Autodesk Inventor part; units mm, degrees
ref_plane "YZ Plane" through (0, 0, 0) normal (1, 0, 0) x (0, 1, 0)
ref_plane "XZ Plane" through (0, 0, 0) normal (0, 1, 0) x (-1, 0, 0)
ref_plane "XY Plane" through (0, 0, 0) normal (0, 0, 1) x (1, 0, 0)
sketch "Sketch1" plane through (0, 0, 0) normal (0, 1, 0) x (-1, 0, 0)
  line L0 (-6.5, -2.5) -> (6.5, -2.5)
  line L1 (6.5, -2.5) -> (6.5, 2.5)
  line L2 (6.5, 2.5) -> (-6.5, 2.5)
  line L3 (-6.5, 2.5) -> (-6.5, -2.5)
  line L4 (-6.5, -2.5) -> (6.5, 2.5) construction
  line L5 (6.5, -2.5) -> (-6.5, 2.5) construction
  point P0 (0, 0)
  dimension "d0" = 13
  dimension "d1" = 5
extrude "Extrusion1" add sketch "Sketch1" along normal blind 70.4
sketch "Sketch2" plane through (0, 70.4, 0) normal (0, 1, 0) x (1, 0, 0)
  line L0 (6.5, 2.5) -> (6.5, -2.5)
  line L1 (6.5, -2.5) -> (-6.5, -2.5)
  line L2 (-6.5, -2.5) -> (-6.5, 2.5)
  line L3 (-6.5, 2.5) -> (6.5, 2.5)
  line L4 (-6.5, -2.5) -> (6.5, -2.5)
  line L5 (6.5, -2.5) -> (6.5, 15.2)
  line L6 (6.5, 15.2) -> (-6.5, 15.2)
  line L7 (-6.5, 15.2) -> (-6.5, -2.5)
  point P0 (0, 0)
  dimension "d4" = 17.7
extrude "Extrusion2" add sketch "Sketch2" against normal blind 5 contours L3 L7 L6 L5
fillet "Fillet1" radius 6.5 2 edges at (6.5, 0, 0) (-6.5, 0, 0)
sketch "Sketch3" plane through (6.5, 65.4, -2.5) normal (0, 0, -1) x (-1, 0, 0)
  arc A0 (0, -58.9) -> (13, -58.9) centre (6.5, -58.9) ccw
  line L0 (0, -58.9) -> (0, 0)
  line L1 (0, 0) -> (0, 5)
  line L2 (0, 5) -> (13, 5)
  line L3 (13, 5) -> (13, 0)
  line L4 (13, 0) -> (13, -58.9)
  line L5 (13, 0) -> (0, 0)
  circle A1 centre (6.5, -58.9) radius 6.5
  point P0 (6.5, -65.4)
extrude "Extrusion3" add sketch "Sketch3" along normal blind 5 contours A1 A0
sketch "Sketch4" plane through (0, 70.4, 0) normal (0, 1, 0) x (1, 0, 0)
  line L0 (6.5, -2.5) -> (-6.5, -2.5)
  line L1 (-6.5, -2.5) -> (-6.5, 15.2)
  line L2 (-6.5, 15.2) -> (6.5, 15.2)
  line L3 (6.5, 15.2) -> (6.5, -2.5)
  line L4 (6.5, -2.5) -> (-6.5, -2.5)
  line L5 (-6.5, -2.5) -> (-6.5, 15.2)
  line L6 (-6.5, 15.2) -> (6.5, 15.2)
  line L7 (6.5, 15.2) -> (6.5, -2.5)
  line L8 (-6.5, 2.5) -> (6.5, 2.5)
  circle A0 centre (0, 8.85) radius 2
  point P0 (0, 0)
  dimension "d10" = 4
  dimension "d11" = 6.35
  dimension "d12" = 6.5
extrude "Extrusion4" cut sketch "Sketch4" against normal up to surface (5 mm away) contours A0
properties part number "terminal_mount_front"
Part model, mm, in its own coordinate system. A direction names the side the tool comes from. Coordinates: 2 decimals unless noted, no trailing zeros. Write each loop counter-clockwise with the first axis right and the second up, starting at its lowest first coordinate (ties: lowest second). Pieces come first, ordered by that corner, then holes. Notation, with made-up numbers: (39.5, 66) - (76.5, 66) arc R30 ccw to (76.5, 90) - close; hole circle Ø1 at (67.25, 28). An arc over 180 degrees is marked (long way). Put each result on its own line as item: value.
1. Band-saw the part on D-D (y = 58.5). Write the cut outline in (x, z), then the cut area to 3 significant figures.
Final values:
outline: (-6.5, -2.5) - (6.5, -2.5) - (6.5, 2.5) - (-6.5, 2.5) - close
area: 65.0 mm²
2. 3-axis set-ups, long thin cutter, end or side, ignore diameter. For faces 1 (the flat face through (-2, 65.4, -10)), 2 (the cylindrical face through (-0.26, 67.935, -10.833)), 3 (the flat face through (0, 7, -7.5)): which of +Z, -Z, +X, -X, +Y, -Y reach the whole face in a straight line?
Final values:
face 1: -Z, +X, -X
face 2: +Y
face 3: -Z, +X, -X, -Y
3. Band-saw the part on B-B (z = -4.75). Write the cut outline in (x, y).
Final values:
outline: circle Ø13 at (0, 6.5); (-6.5, 65.4) - (6.5, 65.4) - (6.5, 70.4) - (-6.5, 70.4) - close
4. Flat gauge pins, fed straight in: pin 1 Ø2 at (x, z) = (0, -11.5) entering from -Y; pin 2 Ø4 at (x, z) = (-3, -6) entering from -Y. Where does each tip first touch, or does it go through?
Final values:
pin 1: stops at y = 65.4
pin 2: stops at y = 0.08
5. Probe line 1 along Z through (x, y) = (0, 68.8); line 2 along X through (y, z) = (66.45, -8.85); line 3 along Z through (x, y) = (-5.5, 50). List the from-to ranges inside material, lowest first. Write a range as [from, to].
Final values:
line 1: z = [-15.2, -10.85], [-6.85, 2.5]
line 2: x = [-6.5, -2], [2, 6.5]
line 3: z = [-2.5, 2.5]
6. Band-saw the part on A-A (z = -8.85). Write the cut outline in (x, y).
Final values:
outline: (-6.5, 65.4) - (-2, 65.4) - (-2, 70.4) - (-6.5, 70.4) - close; (2, 65.4) - (6.5, 65.4) - (6.5, 70.4) - (2, 70.4) - close
7. Two-plate mould, pull along Y, no slides. Class faces 4 (the flat face through (0, 70.4, -6)), 5 (the flat face through (-6.5, 43, -2)), 6 (the flat face through (0, 36, -2.5)): +Y half, -Y half, draft (parallel to the pull), parting line (faces both ways), or undercut.
Final values:
face 4: +Y half
face 5: draft
face 6: undercut
8. Band-saw the part on C-C (x = 3). Write the cut outline in (y, z), then the cut area to 3 significant figures.
Final values:
outline: (0.73, -7.5) - (12.27, -7.5) - (12.27, -2.5) - (65.4, -2.5) - (65.4, -15.2) - (70.4, -15.2) - (70.4, 2.5) - (0.73, 2.5) - close
area: 469 mm²
